Could you check a few things on this model? Use its own coordinates, in mm. Face numbers are marked on the shaded views. A direction names the side the tool comes from. Round coordinates to 2 decimals unless told otherwise and drop trailing zeros. Answer in a Markdown table with one row per item.
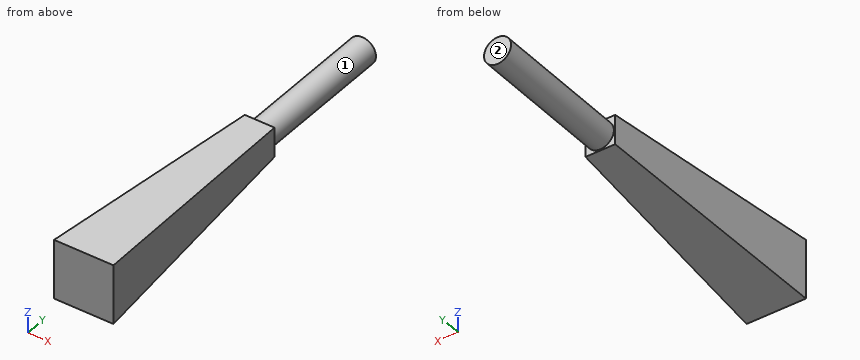
```python
from build123d import *

# Parameters (mm, degrees)
F0_W     = 22
F0_H     = 22
F2_W     = 11
F2_H     = 11
F4_R     = 5.011147
F5_DEPTH = 53


with BuildPart() as f3:
    # F0 (on Front) → F3 section 0
    with BuildSketch(Plane.XZ):
        Rectangle(F0_W, F0_H)
    # F2 (on offset) → F3 section 1
    with BuildSketch(Plane.XZ.offset(-90.7)):
        Rectangle(F2_W, F2_H)
    loft()

    # F4 (on face) → F5 (join)
    with BuildSketch(Plane(origin=(0, 90.7, 0), x_dir=(-1, 0, 0), z_dir=(0, 1, 0))):
        Circle(F4_R)
    extrude(amount=F5_DEPTH)


solid = f3.part
```
1) Which directions (+Z, -Z, +X, -X, +Y, -Y) give clear straight access to the entire face, cutting with the end or side of a thin tool? Please do the marked faces 1 and 2.
Computed:
| item | result |
|---|---|
| face 1 | +Y |
| face 2 | +Z, -Z, +X, -X, +Y |
2) I need wall thicknesses on line 1 (Y direction, x = -3.75, z = 3.75); line 2 (X direction, y = 111, z = 0.5); line 3 (X direction, y = 73, z = -0.25). Which ranges of each line are inside material? Lowest first, please.
Computed:
| item | result |
|---|---|
| line 1 | y = 0 to 90.7 |
| line 2 | x = -4.99 to 4.99 |
| line 3 | x = -6.57 to 6.57 |
3) Will these pins go through, and if not, where does the flat tip stop? P1, Ø1.5, axis at y = 48, z = 4.5, coming from the +X side; P2, Ø1.5, axis at y = 105, z = -3, coming from the -X side; P3, Ø6, axis at x = 2.5, z = -5, coming from the -Y side; P4, Ø2, axis at y = 78.5, z = -1.5, coming from the +X side.
Computed:
| item | result |
|---|---|
| P1 | stops at x = 8.13 |
| P2 | stops at x = -4.48 |
| P3 | stops at y = 0 |
| P4 | stops at x = 6.3 |
